from build123d import *

# Parameters (mm, degrees)
SALIENTE_EXTRUIR1_DEPTH = 88.9
CROQUIS4_R              = 2.999994
CORTAR_EXTRUIR1_DEPTH   = 112.44204772
REDONDEO6_R             = 3
REDONDEO7_R             = 3
ESCALA2_SCALE           = 1.03
SALIENTE_EXTRUIR2_DEPTH = 91.567


with BuildPart() as part:
    # Croquis1 → Saliente-Extruir1 (new body)
    with BuildSketch(Plane(origin=(0, 0, 0), x_dir=(1, 0, 0), z_dir=(0, 1, 0))):
        Polygon((1.696358741, -16.064461222), (13.335, -27.703102481), (0, -50.8), (-13.335, -27.703102481), (-1.696358741, -16.064461222), (-14.760410887, 6.563140847), (-30.659090512, 2.303102481), (-43.994090512, 25.4), (-17.324090512, 25.4), (-13.064052146, 9.501320374), (13.064052146, 9.501320374), (17.324090512, 25.4), (43.994090512, 25.4), (30.659090512, 2.303102481), (14.760410887, 6.563140847), align=None)
    extrude(amount=SALIENTE_EXTRUIR1_DEPTH)

    # Croquis4 → Cortar-Extruir1 (cut, through all)
    with BuildSketch(Plane(origin=(0, 88.9, 0), x_dir=(1, 0, 0), z_dir=(0, 1, 0))):
        with Locations(Location((0, 0, 0), (0, 0, 270))):
            Circle(CROQUIS4_R)
    extrude(amount=-CORTAR_EXTRUIR1_DEPTH, mode=Mode.SUBTRACT)

    # Redondeo6
    redondeo6_edges = [part.edges().sort_by_distance(p)[0] for p in [
        (-1.696358741, 44.45, 16.064461222),
        (-14.760410887, 44.45, -6.563140847),
        (-13.064052146, 44.45, -9.501320374),
        (13.064052146, 44.45, -9.501320374),
        (1.696358741, 44.45, 16.064461222),
    ]]
    fillet(redondeo6_edges, radius=REDONDEO6_R)

    # Redondeo7
    redondeo7_edges = [part.edges().sort_by_distance(p)[0] for p in [
        (-13.335, 44.45, 27.703102481),
        (-30.659090512, 44.45, -2.303102481),
        (-17.324090512, 44.45, -25.4),
        (17.324090512, 44.45, -25.4),
        (30.659090512, 44.45, -2.303102481),
        (13.335, 44.45, 27.703102481),
    ]]
    fillet(redondeo7_edges, radius=REDONDEO7_R)


with BuildPart() as part_1:
    # Escala2: scaled about (-0.008124988, 44.45, 0.003254237)
    add(part.part.scale(ESCALA2_SCALE).moved(Location((0.00024375, -1.3335, -9.7627e-05))))

    # Croquis17 → Saliente-Extruir2 (add, through all)
    with BuildSketch(Plane(origin=(0, 90.2335, 0), x_dir=(1, 0, 0), z_dir=(0, 1, 0))):
        with BuildLine():
            Line((-45.313669478, 56.162097627), (-45.313669478, 26.162097627))
            Line((-45.313669478, 26.162097627), (-40.313669478, 26.162097627))
            Line((-40.313669478, 26.162097627), (-40.313669478, 56.162097627))
            Line((-40.313669478, 56.162097627), (-20.313669478, 56.162097627))
            Line((-20.313669478, 56.162097627), (-20.313669478, 61.162097627))
            Line((-20.313669478, 61.162097627), (-40.313669478, 61.162097627))
            ThreePointArc((-40.313669478, 61.162097627), (-43.849203384, 59.697631533), (-45.313669478, 56.162097627))
        make_face()
        with BuildLine():
            Line((-42.813529111, 21.831727485), (-45.313669478, 26.162097627))
            Line((-45.313669478, 26.162097627), (-71.294291224, 11.161854504))
            ThreePointArc((-71.294291224, 11.161854504), (-73.623920356, 8.125822711), (-73.124418243, 4.331727485))
            Line((-73.124418243, 4.331727485), (-63.124418243, -12.988780591))
            Line((-63.124418243, -12.988780591), (-58.794291224, -10.488780591))
            Line((-58.794291224, -10.488780591), (-68.794291224, 6.831727485))
            Line((-68.794291224, 6.831727485), (-42.813529111, 21.831727485))
        make_face()
        with BuildLine():
            Line((20.313669478, 56.162097627), (40.313669478, 56.162097627))
            Line((40.313669478, 56.162097627), (40.313669478, 26.162097627))
            Line((40.313669478, 26.162097627), (45.313669478, 26.162097627))
            Line((45.313669478, 26.162097627), (45.313669478, 56.162097627))
            ThreePointArc((45.313669478, 56.162097627), (43.849203384, 59.697631533), (40.313669478, 61.162097627))
            Line((40.313669478, 61.162097627), (20.313669478, 61.162097627))
            Line((20.313669478, 61.162097627), (20.313669478, 56.162097627))
        make_face()
        with BuildLine():
            Line((71.294712326, 11.162097627), (45.313669478, 26.162097627))
            Line((45.313669478, 26.162097627), (42.813950212, 21.831970608))
            Line((42.813950212, 21.831970608), (68.794712326, 6.831970608))
            Line((68.794712326, 6.831970608), (58.794712326, -10.488537468))
            Line((58.794712326, -10.488537468), (63.124839345, -12.988537468))
            Line((63.124839345, -12.988537468), (73.124839345, 4.331970608))
            ThreePointArc((73.124839345, 4.331970608), (73.624341457, 8.126065834), (71.294712326, 11.162097627))
        make_face()
        with BuildLine():
            Line((38.481042848, -45.672845092), (28.481042848, -62.993353167))
            Line((28.481042848, -62.993353167), (2.500280734, -47.993353167))
            Line((2.500280734, -47.993353167), (0.000280734, -52.323480186))
            Line((0.000280734, -52.323480186), (25.981042848, -67.323480186))
            ThreePointArc((25.981042848, -67.323480186), (29.775138073, -67.822982299), (32.811169867, -65.493353167))
            Line((32.811169867, -65.493353167), (42.811169867, -48.172845092))
            Line((42.811169867, -48.172845092), (38.481042848, -45.672845092))
        make_face()
        with BuildLine():
            Line((-25.980621746, -67.323723309), (0.000280734, -52.323480186))
            Line((0.000280734, -52.323480186), (-2.499859633, -47.99359629))
            Line((-2.499859633, -47.99359629), (-28.480621746, -62.99359629))
            Line((-28.480621746, -62.99359629), (-38.480621746, -45.673088215))
            Line((-38.480621746, -45.673088215), (-42.810748765, -48.173088215))
            Line((-42.810748765, -48.173088215), (-32.810748765, -65.49359629))
            ThreePointArc((-32.810748765, -65.49359629), (-29.774716972, -67.823225422), (-25.980621746, -67.323723309))
        make_face()
    extrude(amount=-SALIENTE_EXTRUIR2_DEPTH)


solid = part_1.part
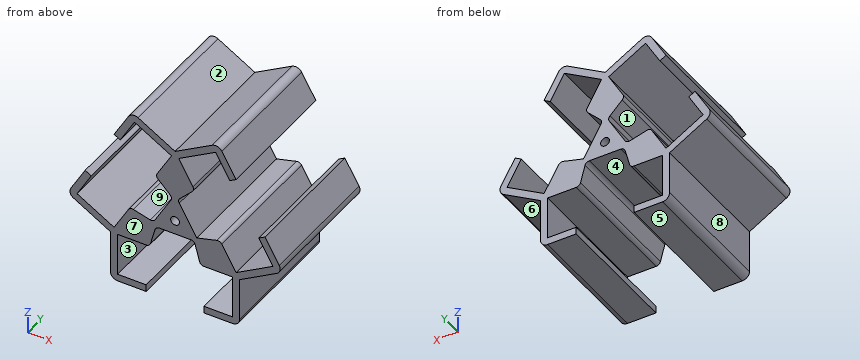
Design review of the part built by this model. Coordinates are the model's own, in mm. Face numbers are marked on the shaded views. A direction names the side the tool comes from. Round coordinates to 2 decimals unless told otherwise and drop trailing zeros. Order: outer loops, then holes, each group sorted by start corner. A loop starts at its lowest first (then second) coordinate and runs counter-clockwise, first axis right, second up. Notation, with made-up numbers: M 78.5,53 L 130.5,53 A11 ccw 130.5,62 Z; hole C 76.25,39 d1. An arc over 180 degrees is marked long. Answer as CSV lines item,"result". Start each with the question number.
1) Add section C-C (z = 55). Give the boundary of the cut face in (x, y).
2) Wall thickness on line 1 along X through (y, z) = (72.5, -48); line 2 along X through (y, z) = (58.5, 60); line 3 along Z through (x, y) = (-4, 68.5): over which ranges is each line inside the solid? List them lowest first. Write a range as [from, to].
3) The part is to be moulded in two halves that separate along X. For the marked faces 6, 7, 8 and 9, say which applies: +X half, -X half, draft (parallel to the pull), parting line (faces both ways), or undercut.
4) Add section D-D (x = 35.5). Give the boundary of the cut face in (y, z).
5) Tool access review of the marked faces 1, 2, 3, 4 and 5: name each direction out of +Z, -Z, +X, -X, +Y, -Y from which nothing blocks a thin tool from reaching the whole face with its end or side.
6) For pin 1 Ø8 at (x, y) = (-3.5, 40) entering from -Z; pin 2 Ø15 at (y, z) = (60.5, -34.5) entering from +X; pin 3 Ø15 at (y, z) = (50, -46.5) entering from -X; pin 4 Ø5 at (x, z) = (-56.5, 14) entering from +Y, all flat-tipped, find the tip position at first contact; note any pin that passes through.
7) Add section B-B (x = -24). Give the boundary of the cut face in (y, z).
8) Add section A-A (z = -42). Give the boundary of the cut face in (x, y), then the cut area to 3 significant figures.
Resolved:
1,outline,"M -38.87,-1.33 L -33.1,-1.33 L -33.1,90.23 L -38.87,90.23 Z; M -14.64,-1.33 L -4.64,-1.33 L -4.64,90.23 L -14.64,90.23 Z; M 4.64,-1.33 L 14.64,-1.33 L 14.64,90.23 L 4.64,90.23 Z; M 33.1,-1.33 L 38.87,-1.33 L 38.87,90.23 L 33.1,90.23 Z"
2,line 1,"[-45.31, -40.31], [40.31, 45.31]"
2,line 2,"[-35.98, -30.21], [-23.3, -13.3], [13.3, 23.3], [30.21, 35.98]"
2,line 3,"[-9.79, 12.64], [18.8, 45.4], [48.86, 54.63]"
3,face 6,"+X half"
3,face 7,"draft"
3,face 8,"-X half"
3,face 9,"undercut"
4,outline,"M -1.33,-61.16 L 90.23,-61.16 L 90.23,-56.16 L -1.33,-56.16 Z; M -1.33,-26.16 L 90.23,-26.16 L 90.23,-9.16 L -1.33,-9.16 Z; M -1.33,50.84 L 90.23,50.84 L 90.23,60.84 L -1.33,60.84 Z"
5,face 1,"-X, +Y, -Y"
5,face 2,"+Z, +Y, -Y"
5,face 3,"+Y, -Y"
5,face 4,"-Z, +Y, -Y"
5,face 5,"-Z, +X, -X, +Y, -Y"
6,pin 1,"z = -9.79"
6,pin 2,"x = 45.31"
6,pin 3,"x = -45.31"
6,pin 4,"through"
7,outline,"M -1.33,-61.16 L 90.23,-61.16 L 90.23,-56.16 L -1.33,-56.16 Z; M -1.33,-26.16 L 90.23,-26.16 L 90.23,-4.4 L -1.33,-4.4 Z; M -1.33,60.41 L 90.23,60.41 L 90.23,66.18 L -1.33,66.18 Z"
8,outline,"M -45.31,-1.33 L -40.31,-1.33 L -40.31,90.23 L -45.31,90.23 Z; M 40.31,-1.33 L 45.31,-1.33 L 45.31,90.23 L 40.31,90.23 Z"
8,area,"916 mm^2"
